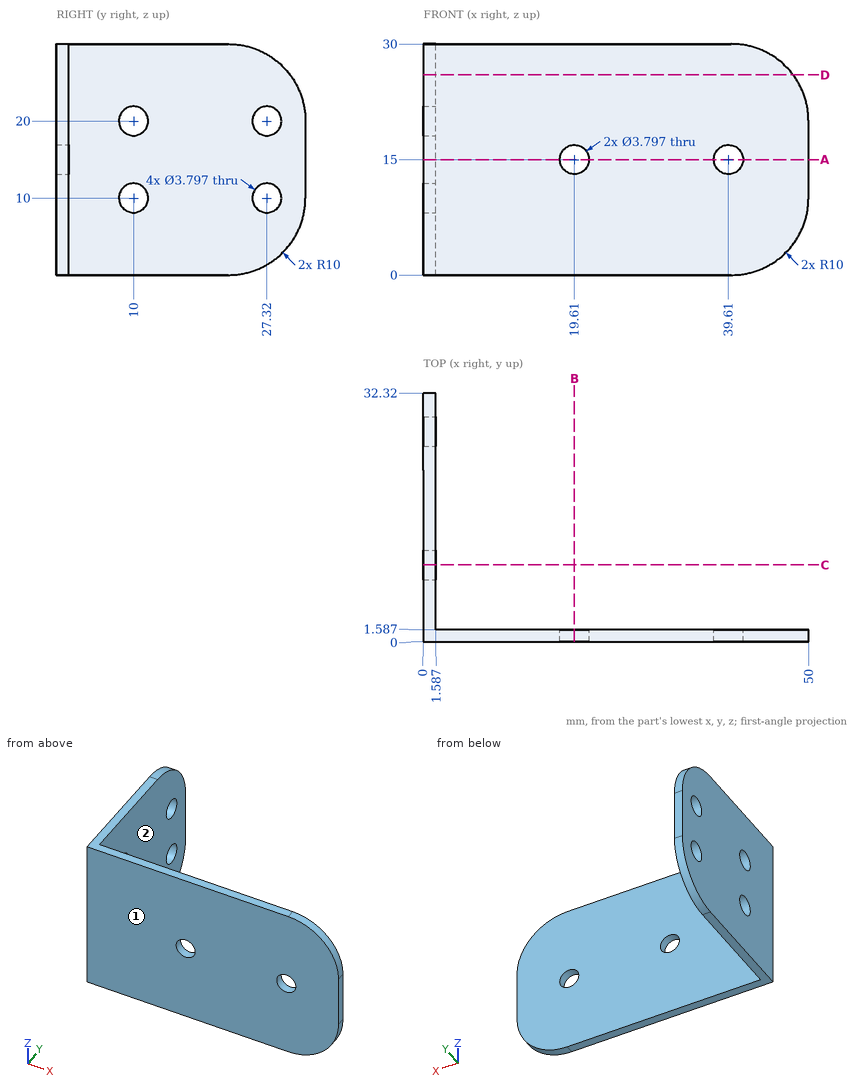
Verification items for this drawing (mm, ordinates from the low corner). A direction names the side the tool comes from. Round coordinates to 2 decimals unless told otherwise and drop trailing zeros. Loops run counter-clockwise (first coordinate to the right, second up) from the corner with the lowest first, then second, coordinate; pieces in that order, holes last. Notation, with made-up numbers: M -38,73.25 L -11,73.25 A26 ccw -11,92.25 Z; hole C 60.25,65.5 d6. An arc over 180 degrees is marked long. Answer as a JSON object with one key per item and string values.
1. Section check A-A (z = 15). Record the boundary of the cut face in (x, y).
Reply:
{"outline": "M 0,0 L 17.71,0 L 17.71,1.59 L 1.59,1.59 L 1.59,32.32 L 0,32.32 Z; M 21.51,0 L 37.71,0 L 37.71,1.59 L 21.51,1.59 Z; M 41.51,0 L 50,0 L 50,1.59 L 41.51,1.59 Z"}
2. Section check C-C (y = 10). Record the boundary of the cut face in (x, z).
Reply:
{"outline": "M 0,0 L 1.59,0 L 1.59,8.1 L 0,8.1 Z; M 0,11.9 L 1.59,11.9 L 1.59,18.1 L 0,18.1 Z; M 0,21.9 L 1.59,21.9 L 1.59,30 L 0,30 Z"}
3. Section check B-B (x = 19.61). Record the boundary of the cut face in (y, z).
Reply:
{"outline": "M 0,0 L 1.59,0 L 1.59,13.1 L 0,13.1 Z; M 0,16.9 L 1.59,16.9 L 1.59,30 L 0,30 Z"}
4. Access from +Z, -Z, +X, -X, +Y, -Y to the whole of each face (thin tool, end or side, straight path). Record for the marked faces 1 and 2.
Reply:
{"face 1": "+Z, -Z, +X, -X, -Y", "face 2": "+Z, -Z, +X, +Y"}
5. Gauge pin test, flat ends, axial feed: P1, Ø2.5, axis at y = 10, z = 20, coming from the -X side; P2, Ø10, axis at x = 31.5, z = 17, coming from the +Y side; P3, Ø10, axis at y = 15, z = 10, coming from the +X side. Record the tip position at first contact, or that the pin passes through.
Reply:
{"P1": "passes through", "P2": "stops at y = 1.59", "P3": "stops at x = 1.59"}
6. Scan lines: line 1 (Y direction, x = 0.95, z = 10); line 2 (Z direction, x = 19.61, y = 0.4); line 3 (Y direction, x = 11, z = 22.5). Record each from-to range of solid material in increasing order.
Reply:
{"line 1": "y = 0 to 8.1, 11.9 to 25.42, 29.22 to 32.32", "line 2": "z = 0 to 13.1, 16.9 to 30", "line 3": "y = 0 to 1.59"}
7. Section check D-D (z = 26). Record the boundary of the cut face in (x, y).
Reply:
{"outline": "M 0,0 L 48,0 L 48,1.59 L 1.59,1.59 L 1.59,30.32 L 0,30.32 Z"}
